from build123d import *

# Parameters (mm, degrees)
SALIENTE_EXTRUIR1_DEPTH = 13
CROQUIS4_W              = 13
CROQUIS4_H              = 45
SALIENTE_EXTRUIR2_DEPTH = 7
CROQUIS5_R              = 2.125
CORTAR_EXTRUIR1_DEPTH   = 160.981248901
CROQUIS6_R              = 4.05
CORTAR_EXTRUIR2_DEPTH   = 5
CORTAR_EXTRUIR3_REACH   = 162.702
CROQUIS7_R              = 2.125
CORTAR_EXTRUIR4_REACH   = 170.702
CORTAR_EXTRUIR4_START   = -8
CROQUIS8_R              = 4.05
REDONDEO2_R             = 10
REDONDEO5_R             = 10


with BuildPart() as part:
    # Croquis1 → Saliente-Extruir1 (new body)
    with BuildSketch(Plane(origin=(0, 0, 0), x_dir=(0, 0, -1), z_dir=(1, 0, 0))):
        Polygon((0, 0), (0, 40), (25, 40), (92, 90.25), (92, 120), (105, 120), (105, 75), (25, 15), (25, 0), align=None)
    extrude(amount=SALIENTE_EXTRUIR1_DEPTH)

    # Croquis4 → Saliente-Extruir2 (add)
    with BuildSketch(Plane(origin=(13, 0, 0), x_dir=(0, 0, -1), z_dir=(1, 0, 0))):
        with Locations((98.5, 97.5)):
            Rectangle(CROQUIS4_W, CROQUIS4_H)
    extrude(amount=SALIENTE_EXTRUIR2_DEPTH)

    # Croquis5 → Cortar-Extruir1 (cut, through all)
    with BuildSketch(Plane(origin=(13, 0, 0), x_dir=(0, 0, -1), z_dir=(1, 0, 0))):
        with Locations((12.5, 30)):
            Circle(CROQUIS5_R)
        with Locations((12.5, 10)):
            Circle(CROQUIS5_R)
    extrude(amount=-CORTAR_EXTRUIR1_DEPTH, mode=Mode.SUBTRACT)

    # Croquis6 → Cortar-Extruir2 (cut)
    with BuildSketch(Plane(origin=(13, 0, 0), x_dir=(0, 0, -1), z_dir=(1, 0, 0))):
        with Locations((12.5, 30)):
            Circle(CROQUIS6_R)
        with Locations((12.5, 10)):
            Circle(CROQUIS6_R)
    extrude(amount=-CORTAR_EXTRUIR2_DEPTH, mode=Mode.SUBTRACT)

    # Croquis7 → Cortar-Extruir3 (cut, up to next)
    with BuildSketch(Plane(origin=(0, 0, -105), x_dir=(-1, 0, 0), z_dir=(0, 0, -1)), mode=Mode.PRIVATE) as cortar_extruir3_sk1:
        with Locations(Location((-10, 110, 0), (0, 0, 90))):
            Circle(CROQUIS7_R)
    cortar_extruir3_tool1 = extrude(cortar_extruir3_sk1.sketch, amount=-CORTAR_EXTRUIR3_REACH, mode=Mode.PRIVATE) & part.part
    # Croquis7 → Cortar-Extruir3 (cut, up to next)
    with BuildSketch(Plane(origin=(0, 0, -105), x_dir=(-1, 0, 0), z_dir=(0, 0, -1)), mode=Mode.PRIVATE) as cortar_extruir3_sk2:
        with Locations(Location((-10, 90, 0), (0, 0, 90))):
            Circle(CROQUIS7_R)
    cortar_extruir3_tool2 = extrude(cortar_extruir3_sk2.sketch, amount=-CORTAR_EXTRUIR3_REACH, mode=Mode.PRIVATE) & part.part
    add(cortar_extruir3_tool1.solids().sort_by_distance((10, 110, -105))[0], mode=Mode.SUBTRACT)
    add(cortar_extruir3_tool2.solids().sort_by_distance((10, 90, -105))[0], mode=Mode.SUBTRACT)

    # Croquis8 → Cortar-Extruir4 (cut, up to next)
    with BuildSketch(Plane(origin=(0, 0, -105), x_dir=(-1, 0, 0), z_dir=(0, 0, -1)).offset(CORTAR_EXTRUIR4_START), mode=Mode.PRIVATE) as cortar_extruir4_sk1:
        with Locations(Location((-10, 110, 0), (0, 0, 90))):
            Circle(CROQUIS8_R)
    cortar_extruir4_tool1 = extrude(cortar_extruir4_sk1.sketch, amount=-CORTAR_EXTRUIR4_REACH, mode=Mode.PRIVATE) & part.part
    # Croquis8 → Cortar-Extruir4 (cut, up to next)
    with BuildSketch(Plane(origin=(0, 0, -105), x_dir=(-1, 0, 0), z_dir=(0, 0, -1)).offset(CORTAR_EXTRUIR4_START), mode=Mode.PRIVATE) as cortar_extruir4_sk2:
        with Locations(Location((-10, 90, 0), (0, 0, 90))):
            Circle(CROQUIS8_R)
    cortar_extruir4_tool2 = extrude(cortar_extruir4_sk2.sketch, amount=-CORTAR_EXTRUIR4_REACH, mode=Mode.PRIVATE) & part.part
    add(cortar_extruir4_tool1.solids().sort_by_distance((10, 110, -97))[0], mode=Mode.SUBTRACT)
    add(cortar_extruir4_tool2.solids().sort_by_distance((10, 90, -97))[0], mode=Mode.SUBTRACT)

    # Redondeo2
    redondeo2_edges = [part.edges().sort_by_distance(p)[0] for p in [
        (6.5, 15, -25),
    ]]
    fillet(redondeo2_edges, radius=REDONDEO2_R)

    # Redondeo5
    # the kernel refuses this fillet: 10 mm, written as the material it adds along each edge
    with BuildSketch(Plane(origin=(0, 40, -25), x_dir=(0, 0, 1), z_dir=(1, 0, 0))) as redondeo5_piece_1:
        with BuildLine():
            CenterArc((REDONDEO5_R * 0.333333333333, -REDONDEO5_R), REDONDEO5_R, 90, 36.869897646)
            Line((-REDONDEO5_R * 0.266666666667, -REDONDEO5_R * 0.2), (0, 0))
            Line((0, 0), (REDONDEO5_R * 0.333333333333, 0))
        make_face()
    extrude(amount=13)
    # the kernel refuses this fillet: 10 mm, written as the material it takes off along each edge
    with BuildSketch(Plane(origin=(-25, 0, 0), x_dir=(0, 0, -1), z_dir=(1, 0, 0)), Plane(origin=(-25, 0, -25), x_dir=(0, 1, 0), z_dir=(1, 0, 0)), Plane(origin=(-25, 40, 0), x_dir=(0, -1, 0), z_dir=(1, 0, 0)), Plane(origin=(20, 120, -130), x_dir=(-1, 0, 0), z_dir=(0, 0, 1))) as redondeo5_2_piece_1:
        with BuildLine():
            CenterArc((REDONDEO5_R, REDONDEO5_R), REDONDEO5_R, 180, 90)
            Line((0, REDONDEO5_R), (0, 0))
            Line((0, 0), (REDONDEO5_R, 0))
        make_face()
    extrude(amount=63, mode=Mode.SUBTRACT)
    with BuildSketch(Plane(origin=(20, 75, -68.151519965), x_dir=(0, 1, 0), z_dir=(0, 0, -1))) as redondeo5_2_piece_2:
        with BuildLine():
            CenterArc((9.539392014, -10), REDONDEO5_R, 90, 72.542396876)
            Line((0, -7), (0, 0))
            Line((0, 0), (9.539392014, 0))
        make_face()
    extrude(amount=60.696960071, mode=Mode.SUBTRACT)
    with BuildSketch(Plane(origin=(0, 120, -67), x_dir=(0, -1, 0), z_dir=(0, 0, -1))) as redondeo5_2_piece_3:
        with BuildLine():
            CenterArc((REDONDEO5_R, -REDONDEO5_R), REDONDEO5_R, 90, 90)
            Line((0, -REDONDEO5_R), (0, 0))
            Line((0, 0), (REDONDEO5_R, 0))
        make_face()
    extrude(amount=63, mode=Mode.SUBTRACT)


solid = part.part
For this review, take the finished solid that the model builds, in its own axes (mm). A direction names the side the tool comes from. Coordinates: 2 decimals unless noted, no trailing zeros. Write each loop counter-clockwise with the first axis right and the second up, starting at its lowest first coordinate (ties: lowest second). Pieces come first, ordered by that corner, then holes. Notation, with made-up numbers: (-38, 47) -> (-13, 47) arc R10 cw to (-13, 58) -> close; hole circle Ø2 at (7.25, 7.5). An arc over 180 degrees is marked (long way). Write each question's results on one line, items separated by ' | '. Start each with the question number.
1) Consider section D-D (x = 17.75). Write out the cut boundary in (y, z).
2) Consider section B-B (z = -12.5). Write out the cut boundary in (x, y) (3 decimals), plus the area to 3 significant figures.
3) Insertion check: pin 1 (4 mm diameter, centred on y = 29, z = -12.5, fed in from +X); pin 2 (10.5 mm diameter, centred on y = 30, z = -12.5, fed in from +X); pin 3 (1 mm diameter, centred on x = 2, z = -36, fed in from -Y) (3 decimals). Each pin has a flat end and moves straight along its axis. Give the tip position at first contact, or say it passes through.
4) Consider section A-A (x = 10). Give the number of separate pieces and of enclosed holes in the cut face, plus the area to 3 significant figures.
5) The part is to be moulded in two halves that separate along Z. For faces 5 (the face through (6.41, 3.01, -2.85)), 6 (the face through (10.535, 26.407, -14.369)), 7 (the face through (13, 43, -44)), say which applies: +Z half, -Z half, draft (parallel to the pull), parting line (faces both ways), or undercut.
6) Consider section C-C (z = -48). Write out the cut boundary in (x, y), plus the area to 3 significant figures.
7) Wall thickness on L1, parallel to Y at x = 3.5, z = -12.5 (3 decimals); L2, parallel to X at y = 110, z = -95; L3, parallel to Z at x = 15, y = 91.5: over which ranges is each line inside the solid? List them lowest first. Write a range as [from, to].
8) For faces 1 (the face through (0, 47, -52)), 2 (the face through (10.54, 8.45, -16.24)), 3 (the face through (10.178, 85.954, -92.857)), 4 (the face through (10, 102, -92)), list the 3-axis set-ups (+Z, -Z, +X, -X, +Y, -Y) from which the entire face can be reached by the end or side of a thin tool; tool diameter is ignored.
Geometry says:
1) outline: (78.22, -105) -> (116.32, -105) -> (116.32, -92) -> (78.22, -92) -> close
2) outline: (0, 0) -> (13, 0) -> (13, 5.95) -> (8, 5.95) -> (8, 7.875) -> (0, 7.875) -> close; (0, 12.125) -> (8, 12.125) -> (8, 14.05) -> (13, 14.05) -> (13, 25.95) -> (8, 25.95) -> (8, 27.875) -> (0, 27.875) -> close; (0, 32.125) -> (8, 32.125) -> (8, 34.05) -> (13, 34.05) -> (13, 40) -> (0, 40) -> close | area: 371 mm^2
3) pin 1: x = 8 | pin 2: x = 13 | pin 3: y = 22.875
4) separate pieces: 3 | enclosed holes: 2 | area: 3,000 mm^2
5) face 5: +Z half | face 6: undercut | face 7: draft
6) outline: (0, 32.25) -> (13, 32.25) -> (13, 57.25) -> (0, 57.25) -> close | area: 325 mm^2
7) L1: [0, 7.875], [12.125, 27.875], [32.125, 40] | L2: [0, 5.95], [14.05, 20] | L3: [-105, -92]
8) face 1: +Z, -Z, -X, +Y, -Y | face 2: +X | face 3: +Z | face 4: +Z, +X, +Y
